from build123d import *

# Parameters (mm, degrees)
SKETCH_1_R          = 2.85
EXTRUDE_1_DEPTH     = 2.2
SKETCH_2_R          = 1.4
EXTRUDE_2_DEPTH     = 10
CHAMFER_1_SIZE      = 0.1
FILLET_1_R          = 0.2
CUT_EXTRUDE_1_DEPTH = 1.5


with BuildPart() as part:
    # Эскиз1 → Бобышка-Вытянуть1 (new body)
    with BuildSketch(Plane(origin=(0, 0, 0), x_dir=(1, 0, 0), z_dir=(0, 1, 0))):
        Circle(SKETCH_1_R)
    extrude(amount=EXTRUDE_1_DEPTH)

    # Эскиз2 → Бобышка-Вытянуть2 (add)
    with BuildSketch(Plane(origin=(0, 2.2, 0), x_dir=(1, 0, 0), z_dir=(0, 1, 0))):
        Circle(SKETCH_2_R)
    extrude(amount=EXTRUDE_2_DEPTH)

    # Фаска1
    chamfer_1_edges = [part.edges().sort_by_distance(p)[0] for p in [
        (-1.4, 12.2, 0),
    ]]
    chamfer(chamfer_1_edges, length=CHAMFER_1_SIZE)

    # Скругление1
    fillet_1_edges = [part.edges().sort_by_distance(p)[0] for p in [
        (-2.85, 0, 0),
        (-2.85, 2.2, 0),
    ]]
    fillet(fillet_1_edges, radius=FILLET_1_R)

    # Эскиз3 → Вырез-Вытянуть1 (cut)
    with BuildSketch(Plane.XZ):
        Polygon((-0.5, 0.5), (-0.5, 2), (0.5, 2), (0.5, 0.5), (2, 0.5), (2, -0.5), (0.5, -0.5), (0.5, -2), (-0.5, -2), (-0.5, -0.5), (-2, -0.5), (-2, 0.5), align=None)
    extrude(amount=-CUT_EXTRUDE_1_DEPTH, mode=Mode.SUBTRACT)


solid = part.part
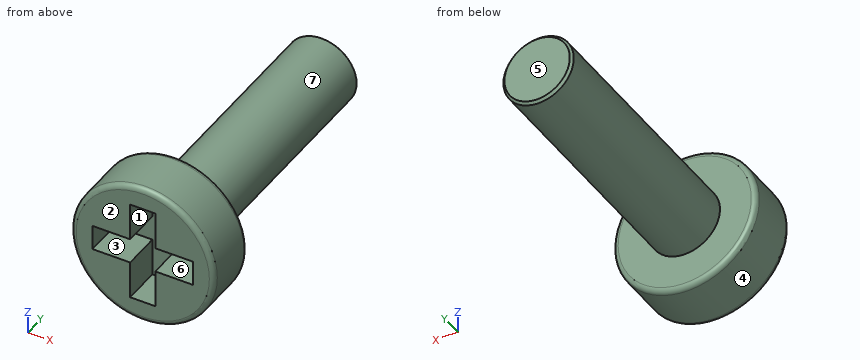
Build history of the part. All positions in model axes, mm. Face numbers are marked on the shaded views. A direction names the side the tool comes from. Give positions to 0.01 mm unless a question says otherwise; leave off trailing zeros. Order: outer loops, then holes, each group sorted by start corner. A loop starts at its lowest first (then second) coordinate and runs counter-clockwise, first axis right, second up. Notation, with made-up numbers: M 16,7.5 L 29,7.5 A18 ccw 29,13.5 Z; hole C 77.5,21.5 d2. An arc over 180 degrees is marked long. Use one line per item in the form item = value.
Q1. Slice it at B-B, the plane z = 0. Write the cut outline in (x, y).
Conclusion:
outline = M -2.85,0.2 A0.2 ccw -2.65,0 L -2,0 L -2,1.5 L 2,1.5 L 2,0 L 2.65,0 A0.2 ccw 2.85,0.2 L 2.85,2 A0.2 ccw 2.65,2.2 L 1.4,2.2 L 1.4,12.1 L 1.3,12.2 L -1.3,12.2 L -1.4,12.1 L -1.4,2.2 L -2.65,2.2 A0.2 ccw -2.85,2 Z
Q2. Slice it at C-C, the plane y = 6.5. Write the cut outline in (x, z), and give its area (3 significant figures).
Conclusion:
outline = C 0,0 d2.8
area = 6.16 mm2
Q3. Which spindle directions (+Z, -Z, +X, -X, +Y, -Y) get a long thin tool onto all of the face, cutting with end or side? Do the marked faces 5, 6 and 7. Say none if no direction does.
Conclusion:
face_5 = +Z, -Z, +X, -X, +Y
face_6 = -Y
face_7 = +Y
Q4. Pull direction Z, two halves, no side cores. Call the marked faces 1, 2, 3 and 4: released by +Z, released by -Z, zero draft, split by the parting line, or undercut.
Conclusion:
face_1 = undercut
face_2 = zero draft
face_3 = undercut
face_4 = split by the parting line
Q5. Wall check: probe 1 along X at (y, z) = (8.5, 0.1); probe 2 along Y at (x, z) = (0.45, -1.55); probe 3 along Y at (x, z) = (-0.1, -0.7). Give the ranges that are in metal, low to high.
Conclusion:
probe_1 = -1.4 to 1.4
probe_2 = 1.5 to 2.2
probe_3 = 1.5 to 12.2
Q6. Pin check, flat tips, straight feed: P1, Ø1.6, axis at y = 1, z = 1, coming from the -X side; P2, Ø0.8, axis at x = -1, y = 1, coming from the +Z side; P3, Ø1.6, axis at y = 0.5, z = 1, coming from the +X side; P4, Ø1, axis at x = 2, y = 10, coming from the +Z side. Stop position of each tip, or through.
Conclusion:
P1 = -2.84
P2 = 2.79
P3 = 2.84
P4 = through
Q7. Slice it at A-A, the plane x = 0. Write the cut outline in (y, z), and give its area (3 significant figures).
Conclusion:
outline = M 0,-2.65 A0.2 ccw 0.2,-2.85 L 2,-2.85 A0.2 ccw 2.2,-2.65 L 2.2,-1.4 L 12.1,-1.4 L 12.2,-1.3 L 12.2,1.3 L 12.1,1.4 L 2.2,1.4 L 2.2,2.65 A0.2 ccw 2,2.85 L 0.2,2.85 A0.2 ccw 0,2.65 L 0,2 L 1.5,2 L 1.5,-2 L 0,-2 Z
area = 34.5 mm2
